Source: CAD feature listing. Evaluate the final solid. Frame: model axes, mm. A direction names the side the tool comes from. Give positions to 0.01 mm unless a question says otherwise; leave off trailing zeros. Order: outer loops, then holes, each group sorted by start corner. A loop starts at its lowest first (then second) coordinate and runs counter-clockwise, first axis right, second up. Notation, with made-up numbers: M 60.5,-35 L 81.5,-35 A16 cw 81.5,-19 Z; hole C 72.5,23 d4. An arc over 180 degrees is marked long. Answer in a Markdown table with one row per item. Add a question column.
(1) Material intervals for line 1 along X through (y, z) = (-0.25, 57) (3 decimals); line 2 along Z through (x, y) = (1, 6); line 3 along Y through (x, z) = (12, 18), sorted ascending.
(2) Section query B-B, the plane x = 0. Return loops of the section in (y, z) (3 decimals).
(3) Pin query (flat end, axial travel): P1, Ø1, axis at x = 0.5, z = 5.5, coming from the +Y side; P2, Ø12, axis at x = 1.5, y = 10, coming from the -Z side; P3, Ø8, axis at x = 14, y = 11, coming from the -Z side; P4, Ø2.5, axis at y = 1.5, z = 19, coming from the -X side. Return the tip coordinate at first contact, or that it passes through.
(4) Set-up query: faces 1 (the face through (16.347, 2.535, -27.61)), 2 (the face through (17.002, 2.465, 57.922)), 3 (the face through (-17, 2, 16)), 4 (the face through (-24, -1, 52.55)). Return all of +Z, -Z, +X, -X, +Y, -Y with unobstructed straight access to the full face (end or side cutting, diameter ignored); none if empty.
(5) Section query D-D, the plane y = 16.5. Return loops of the section in (x, z).
(6) Mould query, pull axis Z, two halves, no side actions, for faces 5 (the face through (-23, -1, 61.45)), 6 (the face through (-16.361, 2.535, 62.593)), 7 (the face through (16.3, 2.54, 62.66)), 8 (the face through (0, 20, -21)). Classes: pulls with the +Z half, pulls with the -Z half, needs draft (parallel to the pull), parting line crosses it, or undercut.
(7) Section query C-C, the plane z = 2. Return loops of the section in (x, y).
Solid Edge part; units mm, degrees
sketch "Sketch1" plane through (0, 0, 0) normal (0, -1, 0) x (1, 0, 0)
  line L0 (-20, 57) -> (-20, -22)
  arc A0 (-20, -22) -> (-10, -32) centre (-10, -22) ccw
  line L1 (-10, -32) -> (10, -32)
  arc A1 (10, -32) -> (20, -22) centre (10, -22) ccw
  line L2 (20, 57) -> (20, -22)
  arc A2 (10, 67) -> (20, 57) centre (10, 57) cw
  line L3 (-10, 67) -> (10, 67)
  arc A3 (-10, 67) -> (-20, 57) centre (-10, 57) ccw
extrude "Protrusion1" add sketch "Sketch1" along normal blind 2
sketch "Sketch2" plane through (0, 0, 0) normal (0, -1, 0) x (1, 0, 0)
  line L0 (17, 56.173) -> (17, -21)
  arc A0 (17, -21) -> (9, -29) centre (9, -21) cw
  line L1 (9, -29) -> (-11, -29)
  arc A1 (-11, -29) -> (-17, -23) centre (-11, -23) cw
  line L2 (-17, -23) -> (-17, 57)
  arc A2 (-17, 57) -> (-10, 64) centre (-10, 57) cw
  line L3 (-10, 64) -> (9.173, 64)
  arc A3 (9.173, 64) -> (17, 56.173) centre (10.0559, 57.0559) cw
extrude "ExtrudedProtrusion_11" add sketch "Sketch2" against normal blind 5
sketch "Sketch3" plane through (0, 0, 0) normal (0, -1, 0) x (1, 0, 0)
  circle A0 centre (0, 19) radius 2.25
  circle A1 centre (0, 38) radius 2.25
  circle A2 centre (0, -21) radius 2.25
extrude "ExtrudedProtrusion_12" add sketch "Sketch3" against normal blind 20
sketch "Sketch4" plane through (0.4, 2, 16.9) normal (0, 1, 0) x (0, 0, 1)
  circle A0 centre (-42.9, 14.1) radius 2.45
  circle A1 centre (-42.9, -14.9) radius 2.45
  circle A2 centre (44.1, -14.9) radius 2.45
  circle A3 centre (44.1, 14.1) radius 2.45
extrude "ExtrudedProtrusion_13" add sketch "Sketch4" along normal blind 3 and the other way blind 4
sketch "Sketch5" plane through (0.4, 0, 16.9) normal (0, -1, 0) x (0, 0, 1)
  circle A0 centre (40.1, 25.3083) radius 2.75
  line L0 (44.55, 29.3083) -> (35.65, 29.3083)
  line L1 (35.65, 29.3083) -> (35.65, 17.4)
  line L2 (35.65, 17.4) -> (44.55, 17.3083)
  line L3 (44.55, 17.3083) -> (44.55, 29.3083)
extrude "ExtrudedProtrusion_18" add sketch "Sketch5" along normal blind 2
sketch "Sketch6" plane through (0, 0, 0) normal (0, -1, 0) x (1, 0, 0)
  circle A0 centre (0, 57) radius 6.995
extrude "ExtrudedCutout_3" cut sketch "Sketch6" along normal mid plane 10
fillet "Round_2" radius 1 2 edges at (-28.9083, -1, 61.45) (-28.9083, -1, 52.55)
Values follow:
| question | item | result |
|---|---|---|
| 1 | line 1 | x = -28.908 to -27.658, -22.158 to -6.995, 6.995 to 20 |
| 1 | line 2 | z = -23.02 to -18.98, 16.98 to 21.02, 35.98 to 40.02 |
| 1 | line 3 | y = -2 to 5 |
| 2 | outline | M -2,-32 L 0,-32 L 0,-29 L 5,-29 L 5,-23.25 L 20,-23.25 L 20,-18.75 L 5,-18.75 L 5,16.75 L 20,16.75 L 20,21.25 L 5,21.25 L 5,35.75 L 20,35.75 L 20,40.25 L 5,40.25 L 5,50.005 L -2,50.005 Z; M -2,63.995 L 5,63.995 L 5,64 L 0,64 L 0,67 L -2,67 Z |
| 3 | P1 | stops at y = 5 |
| 3 | P2 | stops at z = -29 |
| 3 | P3 | passes through |
| 3 | P4 | stops at x = -17 |
| 4 | face 1 | +Y |
| 4 | face 2 | +X, +Y |
| 4 | face 3 | +Z, -Z, -X, +Y |
| 4 | face 4 | -Z, -X, +Y, -Y |
| 5 | outline | C 0,-21 d4.5; C 0,19 d4.5; C 0,38 d4.5 |
| 6 | face 5 | pulls with the +Z half |
| 6 | face 6 | undercut |
| 6 | face 7 | undercut |
| 6 | face 8 | needs draft |
| 7 | outline | M -20,-2 L 20,-2 L 20,0 L 17,0 L 17,5 L -17,5 L -17,0 L -20,0 Z |
